Answer from the drawing. Dimensions are ordinates in mm from the lowest x, y and z of the part. A direction names the side the tool comes from. Coordinates: 2 decimals unless noted, no trailing zeros. Write each loop counter-clockwise with the first axis right and the second up, starting at its lowest first coordinate (ties: lowest second). Pieces come first, ordered by that corner, then holes. Notation, with made-up numbers: (28, -29.5) - (34, -29.5) arc R32 cw to (34, -0.5) - close; hole circle Ø1 at (3, -17). An arc over 180 degrees is marked (long way). Use one line per item in the form item = value. Start each with the question number.
Item 1: A cutting plane is placed at B-B (x = 2). Write down the section's boundary in (y, z).
Item 2: Determine the mould class of the marked faces 1, 2 and 3 for opening direction X: released by +X, released by -X, zero draft, split by the parting line, or undercut.
Item 3: A cutting plane is placed at A-A (z = 4.4). Write down the section's boundary in (x, y), then the cut area to 3 significant figures.
Item 4: Given pin 1 (1 mm diameter, centred on y = 2.5, z = 4, fed in from +X); pin 2 (1.5 mm diameter, centred on x = 15, z = 1, fed in from -Y), each flat-ended and moving along its own axis, determine where each tip first touches the part or whether it passes through.
Item 5: A cutting plane is placed at C-C (z = 0.6). Write down the section's boundary in (x, y).
Item 6: A cutting plane is placed at D-D (y = 14.25). Write down the section's boundary in (x, z).
Item 7: Consider probe 1 along Y at (x, z) = (25.5, 4.65); probe 2 along X at (y, z) = (5.75, 4.2); probe 3 along Z at (x, y) = (6, 11). Determine where each line is inside the solid, lowest interval first.
Item 8: For the marked faces 4, 5 and 6, determine the directions among +Z, -Z, +X, -X, +Y, -Y from which every point of the face is accessible in a straight line to the end or side of a thin tool.
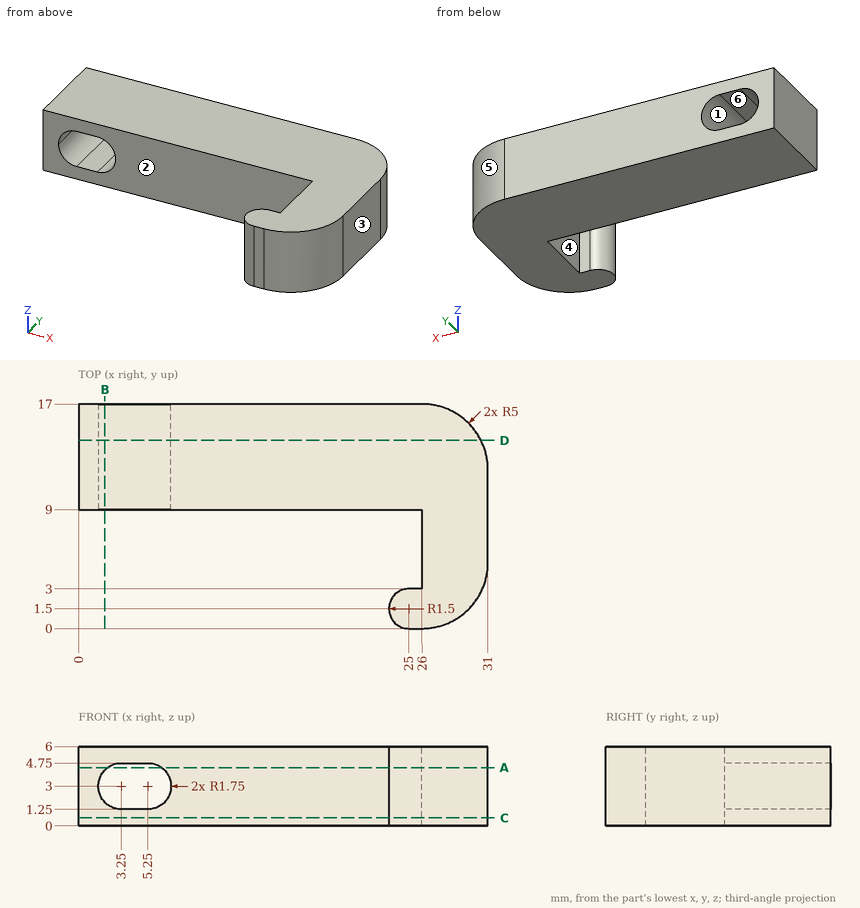
Answer:
q1.outline = (9, 0) - (17, 0) - (17, 1.78) - (9, 1.78) - close; (9, 4.22) - (17, 4.22) - (17, 6) - (9, 6) - close
q2.face_1 = undercut
q2.face_2 = zero draft
q2.face_3 = released by +X
q3.outline = (0, 9) - (2.2, 9) - (2.2, 17) - (0, 17) - close; (6.3, 9) - (26, 9) - (26, 3) - (25, 3) arc R1.5 ccw to (25, 0) - (26, 0) arc R5 ccw to (31, 5) - (31, 12) arc R5 ccw to (26, 17) - (6.3, 17) - close
q3.area = 256 mm²
q4.pin_1 = 30.58
q4.pin_2 = 9
q5.outline = (0, 9) - (26, 9) - (26, 3) - (25, 3) arc R1.5 ccw to (25, 0) - (26, 0) arc R5 ccw to (31, 5) - (31, 12) arc R5 ccw to (26, 17) - (0, 17) - close
q6.outline = (0, 0) - (30.47, 0) - (30.47, 6) - (0, 6) - close; hole (3.25, 1.25) - (5.25, 1.25) arc R1.75 ccw to (5.25, 4.75) - (3.25, 4.75) arc R1.75 ccw to start
q7.probe_1 = 0 to 3, 9 to 17
q7.probe_2 = 26 to 31
q7.probe_3 = 0 to 1.42, 4.58 to 6
q8.face_4 = +Z, -Z, -X
q8.face_5 = +Z, -Z, +X, +Y
q8.face_6 = +Y, -Y
